```python
from build123d import *

# Parameters (mm, degrees)
SKETCH_1_W      = 240
SKETCH_1_H      = 590
SKETCH_1_R      = 21
SKETCH_1_R_2    = 1.75
SKETCH_1_R_3    = 5
SKETCH_1_R_4    = 5.5
SKETCH_1_W_2    = 8
SKETCH_1_H_2    = 30
SKETCH_1_W_3    = 30
SKETCH_1_H_3    = 8
EXTRUDE_1_DEPTH = 5
FILLET_1_R      = 5


with BuildPart() as part:
    # 草图1 → 凸台-拉伸1 (new body)
    with BuildSketch(Plane.XY):
        with Locations((-9.883514394, 97.5)):
            Rectangle(SKETCH_1_W, SKETCH_1_H)
        with Locations((70.116485606, 367.5)):
            Circle(SKETCH_1_R, mode=Mode.SUBTRACT)
        with Locations((70.116485606, 97.5)):
            Circle(SKETCH_1_R, mode=Mode.SUBTRACT)
        with Locations((70.116485606, -172.5)):
            Circle(SKETCH_1_R, mode=Mode.SUBTRACT)
        with Locations((-89.883514394, 367.5)):
            Circle(SKETCH_1_R, mode=Mode.SUBTRACT)
        with Locations((-89.883514394, 97.5)):
            Circle(SKETCH_1_R, mode=Mode.SUBTRACT)
        with Locations((-89.883514394, -172.5)):
            Circle(SKETCH_1_R, mode=Mode.SUBTRACT)
        with Locations((-109.883514394, 275.954136104)):
            Circle(SKETCH_1_R_2, mode=Mode.SUBTRACT)
        with Locations((-79.883514394, 275.954136104)):
            Circle(SKETCH_1_R_2, mode=Mode.SUBTRACT)
        with Locations((-49.883514394, 275.954136104)):
            Circle(SKETCH_1_R_2, mode=Mode.SUBTRACT)
        with Locations((-19.883514394, 275.954136104)):
            Circle(SKETCH_1_R_2, mode=Mode.SUBTRACT)
        with Locations((10.116485606, 275.954136104)):
            Circle(SKETCH_1_R_2, mode=Mode.SUBTRACT)
        with Locations((40.116485606, 275.954136104)):
            Circle(SKETCH_1_R_2, mode=Mode.SUBTRACT)
        with Locations((40.116485606, 199.045863896)):
            Circle(SKETCH_1_R_2, mode=Mode.SUBTRACT)
        with Locations((10.116485606, 199.045863896)):
            Circle(SKETCH_1_R_2, mode=Mode.SUBTRACT)
        with Locations((-19.883514394, 199.045863896)):
            Circle(SKETCH_1_R_2, mode=Mode.SUBTRACT)
        with Locations((-49.883514394, 199.045863896)):
            Circle(SKETCH_1_R_2, mode=Mode.SUBTRACT)
        with Locations((-109.883514394, 199.045863896)):
            Circle(SKETCH_1_R_2, mode=Mode.SUBTRACT)
        with Locations((-79.883514394, 199.045863896)):
            Circle(SKETCH_1_R_2, mode=Mode.SUBTRACT)
        with Locations((70.116485606, 275.954136104)):
            Circle(SKETCH_1_R_2, mode=Mode.SUBTRACT)
        with Locations((70.116485606, 199.045863896)):
            Circle(SKETCH_1_R_2, mode=Mode.SUBTRACT)
        with Locations((40.116485606, -80.954136104)):
            Circle(SKETCH_1_R_2, mode=Mode.SUBTRACT)
        with Locations((10.116485606, -80.954136104)):
            Circle(SKETCH_1_R_2, mode=Mode.SUBTRACT)
        with Locations((-19.883514394, -80.954136104)):
            Circle(SKETCH_1_R_2, mode=Mode.SUBTRACT)
        with Locations((-49.883514394, -80.954136104)):
            Circle(SKETCH_1_R_2, mode=Mode.SUBTRACT)
        with Locations((-79.883514394, -80.954136104)):
            Circle(SKETCH_1_R_2, mode=Mode.SUBTRACT)
        with Locations((-109.883514394, -80.954136104)):
            Circle(SKETCH_1_R_2, mode=Mode.SUBTRACT)
        with Locations((70.116485606, -4.045863896)):
            Circle(SKETCH_1_R_2, mode=Mode.SUBTRACT)
        with Locations((-79.883514394, -4.045863896)):
            Circle(SKETCH_1_R_2, mode=Mode.SUBTRACT)
        with Locations((-109.883514394, -4.045863896)):
            Circle(SKETCH_1_R_2, mode=Mode.SUBTRACT)
        with Locations((-49.883514394, -4.045863896)):
            Circle(SKETCH_1_R_2, mode=Mode.SUBTRACT)
        with Locations((-19.883514394, -4.045863896)):
            Circle(SKETCH_1_R_2, mode=Mode.SUBTRACT)
        with Locations((10.116485606, -4.045863896)):
            Circle(SKETCH_1_R_2, mode=Mode.SUBTRACT)
        with Locations((40.116485606, -4.045863896)):
            Circle(SKETCH_1_R_2, mode=Mode.SUBTRACT)
        with Locations((70.116485606, -80.954136104)):
            Circle(SKETCH_1_R_2, mode=Mode.SUBTRACT)
        with Locations((0.12170833, 345.137685343)):
            Circle(SKETCH_1_R_3, mode=Mode.SUBTRACT)
        with Locations((0.12170833, 75.137685343)):
            Circle(SKETCH_1_R_3, mode=Mode.SUBTRACT)
        with Locations((-6.399865329, -149.662314657)):
            Circle(SKETCH_1_R_4, mode=Mode.SUBTRACT)
        with BuildLine():
            Line((-48.233514394, 337.471968803), (-18.533514394, 337.471968803))
            ThreePointArc((-18.533514394, 337.471968803), (-16.391378464, 335.329832872), (-18.533514394, 333.187696941))
            Line((-18.533514394, 333.187696941), (-48.233514394, 333.187696941))
            ThreePointArc((-48.233514394, 333.187696941), (-50.375650325, 335.329832872), (-48.233514394, 337.471968803))
        make_face(mode=Mode.SUBTRACT)
        with BuildLine():
            Line((-48.233514394, 307.455426815), (-18.533514394, 307.455426815))
            ThreePointArc((-18.533514394, 307.455426815), (-16.407920452, 305.329832872), (-18.533514394, 303.20423893))
            Line((-18.533514394, 303.20423893), (-48.233514394, 303.20423893))
            ThreePointArc((-48.233514394, 303.20423893), (-50.359108337, 305.329832872), (-48.233514394, 307.455426815))
        make_face(mode=Mode.SUBTRACT)
        with BuildLine():
            Line((10.016314713, 325.85), (10.016314713, 296.15))
            ThreePointArc((10.016314713, 296.15), (7.887416749, 294.021102036), (5.758518785, 296.15))
            Line((5.758518785, 296.15), (5.758518785, 325.85))
            ThreePointArc((5.758518785, 325.85), (7.887416749, 327.978897964), (10.016314713, 325.85))
        make_face(mode=Mode.SUBTRACT)
        with BuildLine():
            Line((40.045683981, 325.85), (40.045683981, 296.15))
            ThreePointArc((40.045683981, 296.15), (37.887416749, 293.991732767), (35.729149516, 296.15))
            Line((35.729149516, 296.15), (35.729149516, 325.85))
            ThreePointArc((35.729149516, 325.85), (37.887416749, 328.008267233), (40.045683981, 325.85))
        make_face(mode=Mode.SUBTRACT)
        with BuildLine():
            Line((-48.233514394, 161.804708914), (-18.533514394, 161.804708914))
            ThreePointArc((-18.533514394, 161.804708914), (-16.345684038, 159.616878557), (-18.533514394, 157.429048201))
            Line((-18.533514394, 157.429048201), (-48.233514394, 157.429048201))
            ThreePointArc((-48.233514394, 157.429048201), (-50.421344751, 159.616878557), (-48.233514394, 161.804708914))
        make_face(mode=Mode.SUBTRACT)
        with BuildLine():
            Line((-48.233514394, 131.781482951), (-18.533514394, 131.781482951))
            ThreePointArc((-18.533514394, 131.781482951), (-16.368910001, 129.616878557), (-18.533514394, 127.452274164))
            Line((-18.533514394, 127.452274164), (-48.233514394, 127.452274164))
            ThreePointArc((-48.233514394, 127.452274164), (-50.398118788, 129.616878557), (-48.233514394, 131.781482951))
        make_face(mode=Mode.SUBTRACT)
        with BuildLine():
            Line((9.950676084, 168.85), (9.950676084, 139.15))
            ThreePointArc((9.950676084, 139.15), (7.780411189, 136.979735105), (5.610146295, 139.15))
            Line((5.610146295, 139.15), (5.610146295, 168.85))
            ThreePointArc((5.610146295, 168.85), (7.780411189, 171.020264895), (9.950676084, 168.85))
        make_face(mode=Mode.SUBTRACT)
        with BuildLine():
            Line((39.949177668, 168.85), (39.949177668, 139.15))
            ThreePointArc((39.949177668, 139.15), (37.780411189, 136.981233521), (35.611644711, 139.15))
            Line((35.611644711, 139.15), (35.611644711, 168.85))
            ThreePointArc((35.611644711, 168.85), (37.780411189, 171.018766479), (39.949177668, 168.85))
        make_face(mode=Mode.SUBTRACT)
        with BuildLine():
            Line((5.630411189, -104.15), (5.630411189, -133.85))
            ThreePointArc((5.630411189, -133.85), (7.780411189, -136), (9.930411189, -133.85))
            Line((9.930411189, -133.85), (9.930411189, -104.15))
            ThreePointArc((9.930411189, -104.15), (7.780411189, -102), (5.630411189, -104.15))
        make_face(mode=Mode.SUBTRACT)
        with BuildLine():
            Line((35.630411189, -104.15), (35.630411189, -133.85))
            ThreePointArc((35.630411189, -133.85), (37.780411189, -136), (39.930411189, -133.85))
            Line((39.930411189, -133.85), (39.930411189, -104.15))
            ThreePointArc((39.930411189, -104.15), (37.780411189, -102), (35.630411189, -104.15))
        make_face(mode=Mode.SUBTRACT)
        with BuildLine():
            Line((-48.233514394, -108.162604787), (-18.533514394, -108.162604787))
            ThreePointArc((-18.533514394, -108.162604787), (-16.412712465, -110.283406716), (-18.533514394, -112.404208645))
            Line((-18.533514394, -112.404208645), (-48.233514394, -112.404208645))
            ThreePointArc((-48.233514394, -112.404208645), (-50.354316324, -110.283406716), (-48.233514394, -108.162604787))
        make_face(mode=Mode.SUBTRACT)
        with BuildLine():
            Line((-48.233514394, -138.079324724), (-18.533514394, -138.079324724))
            ThreePointArc((-18.533514394, -138.079324724), (-16.329432402, -140.283406716), (-18.533514394, -142.487488708))
            Line((-18.533514394, -142.487488708), (-48.233514394, -142.487488708))
            ThreePointArc((-48.233514394, -142.487488708), (-50.437596387, -140.283406716), (-48.233514394, -138.079324724))
        make_face(mode=Mode.SUBTRACT)
        with Locations((-89.883514394, 144.5)):
            Rectangle(SKETCH_1_W_2, SKETCH_1_H_2, mode=Mode.SUBTRACT)
        with Locations((23.116485606, 97.5)):
            Rectangle(SKETCH_1_W_3, SKETCH_1_H_3, mode=Mode.SUBTRACT)
        with Locations((-89.883514394, 320.5)):
            Rectangle(SKETCH_1_W_2, SKETCH_1_H_2, mode=Mode.SUBTRACT)
        with Locations((-89.883514394, -125.5)):
            Rectangle(SKETCH_1_W_2, SKETCH_1_H_2, mode=Mode.SUBTRACT)
        with Locations((23.116485606, -172.5)):
            Rectangle(SKETCH_1_W_3, SKETCH_1_H_3, mode=Mode.SUBTRACT)
        with Locations((23.116485606, 367.5)):
            Rectangle(SKETCH_1_W_3, SKETCH_1_H_3, mode=Mode.SUBTRACT)
        with BuildLine():
            Line((60.116485606, -32.5), (60.116485606, -52.5))
            ThreePointArc((60.116485606, -52.5), (57.187553417, -59.571067812), (50.116485606, -62.5))
            Line((50.116485606, -62.5), (-69.883514394, -62.5))
            ThreePointArc((-69.883514394, -62.5), (-76.954582206, -59.571067812), (-79.883514394, -52.5))
            Line((-79.883514394, -52.5), (-79.883514394, -32.5))
            ThreePointArc((-79.883514394, -32.5), (-76.954582206, -25.428932188), (-69.883514394, -22.5))
            Line((-69.883514394, -22.5), (50.116485606, -22.5))
            ThreePointArc((50.116485606, -22.5), (57.187553417, -25.428932188), (60.116485606, -32.5))
        make_face(mode=Mode.SUBTRACT)
        with BuildLine():
            Line((50.116485606, 217.5), (-69.883514394, 217.5))
            ThreePointArc((-69.883514394, 217.5), (-76.954582206, 220.428932188), (-79.883514394, 227.5))
            Line((-79.883514394, 227.5), (-79.883514394, 247.5))
            ThreePointArc((-79.883514394, 247.5), (-76.954582206, 254.571067812), (-69.883514394, 257.5))
            Line((-69.883514394, 257.5), (50.116485606, 257.5))
            ThreePointArc((50.116485606, 257.5), (57.187553417, 254.571067812), (60.116485606, 247.5))
            Line((60.116485606, 247.5), (60.116485606, 227.5))
            ThreePointArc((60.116485606, 227.5), (57.187553417, 220.428932188), (50.116485606, 217.5))
        make_face(mode=Mode.SUBTRACT)
    extrude(amount=EXTRUDE_1_DEPTH)

    # 圆角1
    fillet_1_edges = [part.edges().sort_by_distance(p)[0] for p in [
        (-129.883514394, 392.5, 2.5),
        (110.116485606, 392.5, 2.5),
        (110.116485606, -197.5, 2.5),
        (-129.883514394, -197.5, 2.5),
    ]]
    fillet(fillet_1_edges, radius=FILLET_1_R)


solid = part.part
```
Can you work these out from the model? Positions are in its coordinate system, mm. A direction names the side the tool comes from. Give positions to 0.01 mm unless a question says otherwise; leave off trailing zeros. Write each loop counter-clockwise with the first axis right and the second up, starting at its lowest first coordinate (ties: lowest second). Pieces come first, ordered by that corner, then holes. Notation, with made-up numbers: (48, -29.5) - (52, -29.5) arc R22 ccw to (52, -11.5) - close; hole circle Ø3 at (70.5, 19). An arc over 180 degrees is marked (long way). Write item = value, one per line. Start each with the question number.
1. Thinking about a two-plate mould opening in Y: for faces 1 (the face through (67.38, 388.32, 2.46)), 2 (the face through (-76.876, 220.352, 2.465)), 3 (the face through (-12, 102, 5)), which applies, released by +Y, released by -Y, zero draft, split by the parting line, or undercut?
2. Imagine slicing it at B-B (z = 2). Count the separate pieces of the cut face and the enclosed holes in it, and give its area (3 significant figures).
3. Imagine slicing it at A-A (x = 24). Please give me the cut outline in (y, z), and give its area (3 significant figures).
4. On a 3-axis mill with a long thin cutter (end or side, diameter ignored), from which of +Z, -Z, +X, -X, +Y, -Y can I reach the whole of each face in a straight line? I mean faces 4 (the face through (-12, 102, 0)), 5 (the face through (-76.876, -59.648, 2.465)). Say none if no direction works.
5. Please list where these lines run through material, in increasing order: line 1 (Y direction, x = 14.5, z = 3); line 2 (X direction, y = 326.5, z = 1.1); line 3 (X direction, y = 160, z = 2.7).
Worked answers:
q1.face_1 = undercut
q1.face_2 = undercut
q1.face_3 = zero draft
q2.separate_pieces = 1
q2.enclosed_holes = 57
q2.area = 119,000 mm2
q3.outline = (-197.5, 0) - (-176.5, 0) - (-176.5, 5) - (-197.5, 5) - close; (-168.5, 0) - (-62.5, 0) - (-62.5, 5) - (-168.5, 5) - close; (-22.5, 0) - (93.5, 0) - (93.5, 5) - (-22.5, 5) - close; (101.5, 0) - (217.5, 0) - (217.5, 5) - (101.5, 5) - close; (257.5, 0) - (363.5, 0) - (363.5, 5) - (257.5, 5) - close; (371.5, 0) - (392.5, 0) - (392.5, 5) - (371.5, 5) - close
q3.area = 2,430 mm2
q4.face_4 = -Z, +X, -X, +Y, -Y
q4.face_5 = +Z, -Z
q5.line_1 = -197.5 to -176.5, -168.5 to -62.5, -22.5 to 93.5, 101.5 to 217.5, 257.5 to 363.5, 371.5 to 392.5
q5.line_2 = -129.88 to -93.88, -85.88 to 5.86, 9.91 to 35.83, 39.95 to 110.12
q5.line_3 = -129.88 to -50.39, -16.38 to 5.61, 9.95 to 35.61, 39.95 to 110.12
